```python
from build123d import *
from build123d.topology import SkipClean

# Parameters (mm, degrees)
SKETCH1_R           = 2.55
BOSS_EXTRUDE2_DEPTH = 6
SKETCH7_W           = 32
SKETCH7_H           = 44
BOSS_EXTRUDE3_DEPTH = 6
FILLET1_R           = 2.5
SKETCH3_R           = 7.975
CUT_EXTRUDE2_DEPTH  = 49.602983448
SKETCH2_R           = 1.55
CUT_EXTRUDE1_DEPTH  = 49.602983448
SKETCH6_W           = 60
SKETCH6_H           = 50
CUT_EXTRUDE5_DEPTH  = 1
SKETCH8_R           = 3
CUT_EXTRUDE6_DEPTH  = 4
SKETCH9_R           = 2.55
CUT_EXTRUDE7_DEPTH  = 49.602983448


with BuildPart() as part:
    # Sketch1 → Boss-Extrude2 (new body)
    with BuildSketch(Plane.XY):
        with BuildLine():
            Line((-10, -15), (-10, 15))
            Line((-10, 15), (-15, 30))
            ThreePointArc((-15, 30), (0, 45), (15, 30))
            Line((15, 30), (10, 15))
            Line((10, 15), (10, -15))
            Line((10, -15), (-10, -15))
        make_face()
        Circle(SKETCH1_R, mode=Mode.SUBTRACT)
        with Locations((0, -10)):
            Circle(SKETCH1_R, mode=Mode.SUBTRACT)
    extrude(amount=BOSS_EXTRUDE2_DEPTH)

    # Sketch7 → Boss-Extrude3 (add)
    with BuildSketch(Plane(origin=(0, 0, 0), x_dir=(-1, 0, 0), z_dir=(0, 0, -1))):
        with Locations((0, 23.5)):
            Rectangle(SKETCH7_W, SKETCH7_H)
    extrude(amount=-BOSS_EXTRUDE3_DEPTH)

    # Fillet1
    fillet1_edges = [part.edges().sort_by_distance(p)[0] for p in [
        (10, -15, 3),
        (-10, -15, 3),
        (-16, 1.5, 3),
        (-10, 1.5, 3),
        (10, 1.5, 3),
        (16, 1.5, 3),
        (16, 45.5, 3),
        (-16, 45.5, 3),
    ]]
    fillet(fillet1_edges, radius=FILLET1_R)

    # Sketch3 → Cut-Extrude2 (cut, through all)
    with BuildSketch(Plane.XY.offset(6)):
        with Locations((0, 30)):
            Circle(SKETCH3_R)
    extrude(amount=-CUT_EXTRUDE2_DEPTH, mode=Mode.SUBTRACT)

    # Sketch2 → Cut-Extrude1 (cut, through all)
    with BuildSketch(Plane.XY.offset(6)):
        with Locations((-9, 39)):
            Circle(SKETCH2_R)
        with Locations((9, 39)):
            Circle(SKETCH2_R)
        with Locations((9, 6)):
            Circle(SKETCH2_R)
        with Locations((-9, 6)):
            Circle(SKETCH2_R)
    extrude(amount=-CUT_EXTRUDE1_DEPTH, mode=Mode.SUBTRACT)

    # Sketch6 → Cut-Extrude5 (cut)
    with BuildSketch(Plane.XY.offset(6)):
        with Locations((0, 30)):
            Rectangle(SKETCH6_W, SKETCH6_H)
    extrude(amount=-CUT_EXTRUDE5_DEPTH, mode=Mode.SUBTRACT)

    # Sketch8 → Cut-Extrude6 (cut)
    with BuildSketch(Plane.XY.offset(6)):
        with Locations((-9, 39)):
            Circle(SKETCH8_R)
        with Locations((9, 39)):
            Circle(SKETCH8_R)
        with Locations((9, 6)):
            Circle(SKETCH8_R)
        with Locations((-9, 6)):
            Circle(SKETCH8_R)
    extrude(amount=-CUT_EXTRUDE6_DEPTH, mode=Mode.SUBTRACT)

    # Sketch9 → Cut-Extrude7 (cut, through all)
    with SkipClean():  # the faces are left unmerged after this step: merging them gives an invalid solid
        with BuildSketch(Plane.XY.offset(6)):
            with Locations((0, -10)):
                Circle(SKETCH9_R)
            Circle(SKETCH9_R)
        extrude(amount=-CUT_EXTRUDE7_DEPTH, mode=Mode.SUBTRACT)


solid = part.part
```
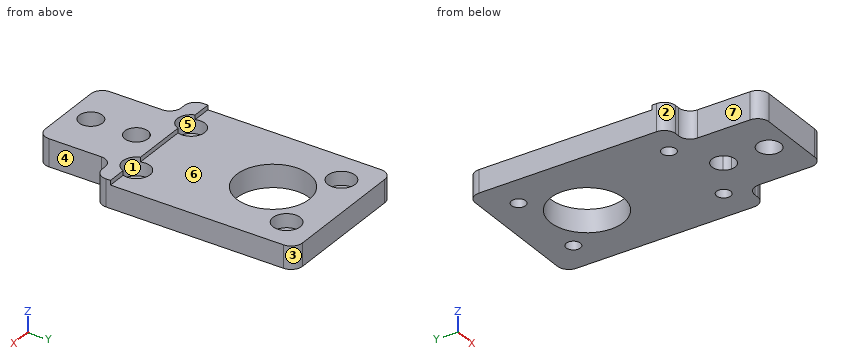
Here's how the part is built. I have some questions about the finished solid (model axes, mm). Face numbers are marked on the shaded views. A direction names the side the tool comes from. Coordinates: 2 decimals unless noted, no trailing zeros. Order: outer loops, then holes, each group sorted by start corner. A loop starts at its lowest first (then second) coordinate and runs counter-clockwise, first axis right, second up. Notation, with made-up numbers: (-34, 71) - (-6, 71) arc R31 cw to (-6, 104) - close; hole circle Ø10 at (32.25, -9.5). An arc over 180 degrees is marked (long way). One line per question, with ' | ' between items. Start each with the question number.
1. If we section it at B-B (z = 1.2): Write out the boundary of the cut face in (x, y) (3 decimals), and give its area (3 significant figures).
2. Please list where these lines run through material, in increasing order: line 1 along X through (y, z) = (6, 4.85); line 2 along Y through (x, z) = (9, 4.1); line 3 along Y through (x, z) = (9, 1.15). Write a range as [from, to].
3. If we section it at A-A (x = 0): Write out the boundary of the cut face in (y, z) (3 decimals), and give its area (3 significant figures).
4. I'm going to push flat-ended pins straight in: pin 1 Ø4 at (x, y) = (-8.5, 14.5) entering from -Z; pin 2 Ø5 at (x, y) = (-9, 39) entering from +Z; pin 3 Ø3 at (x, y) = (9, 39) entering from -Z; pin 4 Ø0.8 at (x, z) = (-3, 5.5) entering from +Y. Where does each tip first touch, or does it pass through?
5. If we section it at C-C (y = -10): Write out the boundary of the cut face in (x, z), and give its area (3 significant figures).
6. If we mould it in two halves opening along X, with no side actions, what happens to the marked faces 1, 2 and 3? For each: released by +X, released by -X, zero draft, split by the parting line, or undercut.
7. Which directions (+Z, -Z, +X, -X, +Y, -Y) give clear straight access to the entire face, cutting with the end or side of a thin tool? Please do the marked faces 4, 5, 6 and 7.
8. If we section it at D-D (y = 39): Write out the boundary of the cut face in (x, z), and give its area (3 significant figures).
Model answer:
1) outline: (-16, 4) arc R2.5 ccw to (-13.5, 1.5) - (-12.5, 1.5) arc R2.5 cw to (-10, -1) - (-10, -12.5) arc R2.5 ccw to (-7.5, -15) - (7.5, -15) arc R2.5 ccw to (10, -12.5) - (10, -1) arc R2.5 cw to (12.5, 1.5) - (13.5, 1.5) arc R2.5 ccw to (16, 4) - (16, 43) arc R2.5 ccw to (13.5, 45.5) - (-13.5, 45.5) arc R2.5 ccw to (-16, 43) - close; hole circle Ø3.1 at (-9, 6); hole circle Ø3.1 at (-9, 39); hole circle Ø15.95 at (0, 30); hole circle Ø5.1 at (0, -10); hole circle Ø5.1 at (0, 0); hole circle Ø3.1 at (9, 6); hole circle Ø3.1 at (9, 39) | area: 1,460 mm²
2) line 1: x = [-16, -12], [-6, 6], [12, 16] | line 2: y = [-14.5, 3], [9, 36], [42, 45.5] | line 3: y = [-14.5, 4.45], [7.55, 37.45], [40.55, 45.5]
3) outline: (-15, 0) - (-12.55, 0) - (-12.55, 6) - (-15, 6) - close; (-7.45, 0) - (-2.55, 0) - (-2.55, 6) - (-7.45, 6) - close; (2.55, 0) - (22.025, 0) - (22.025, 5) - (5, 5) - (5, 6) - (2.55, 6) - close; (37.975, 0) - (45.5, 0) - (45.5, 5) - (37.975, 5) - close | area: 182 mm²
4) pin 1: stops at z = 0 | pin 2: stops at z = 2 | pin 3: passes through | pin 4: stops at y = 5
5) outline: (-10, 0) - (-2.55, 0) - (-2.55, 6) - (-10, 6) - close; (2.55, 0) - (10, 0) - (10, 6) - (2.55, 6) - close | area: 89.4 mm²
6) face 1: undercut | face 2: released by -X | face 3: released by +X
7) face 4: +Z, -Z, +X, -Y | face 5: +Z | face 6: +Z, +X, -X, +Y | face 7: +Z, -Z, -X, -Y
8) outline: (-16, 0) - (-10.55, 0) - (-10.55, 2) - (-12, 2) - (-12, 5) - (-16, 5) - close; (-7.45, 0) - (7.45, 0) - (7.45, 2) - (6, 2) - (6, 5) - (-6, 5) - (-6, 2) - (-7.45, 2) - close; (10.55, 0) - (16, 0) - (16, 5) - (12, 5) - (12, 2) - (10.55, 2) - close | area: 112 mm²
